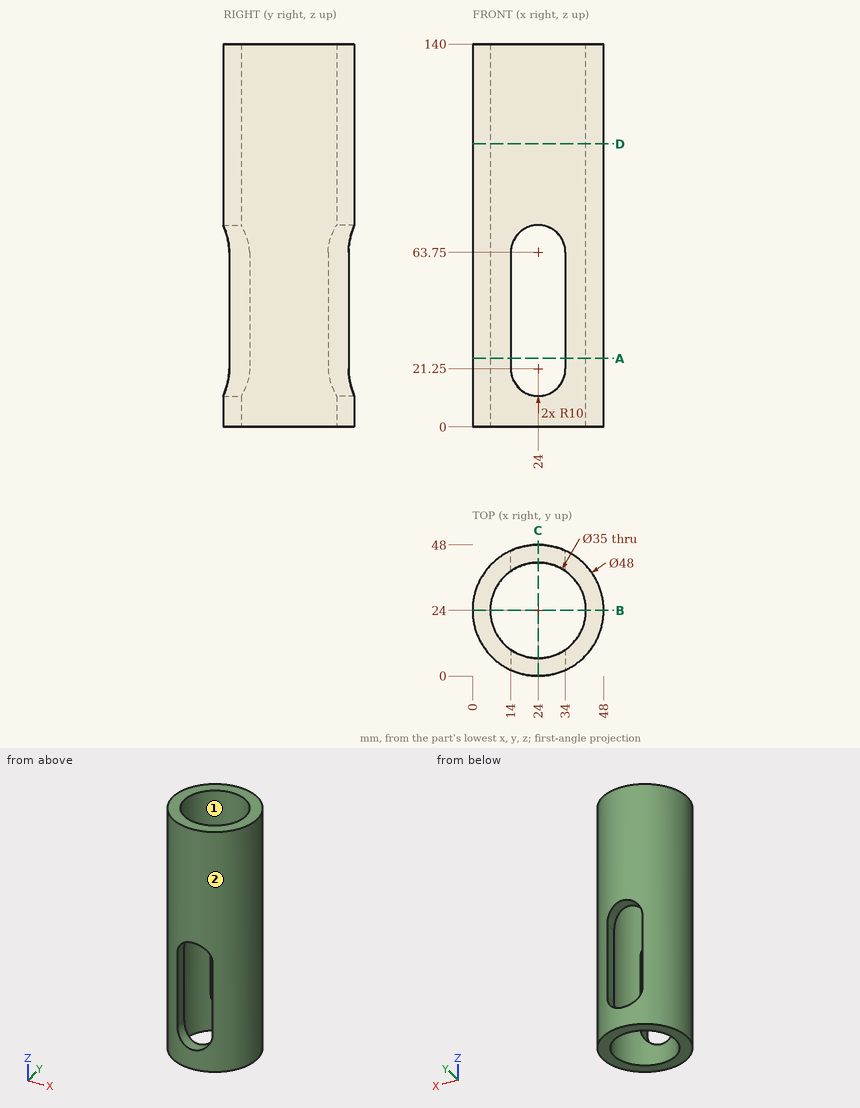
The figure shows three views and two pictorial views of one solid part (mm, origin at its lowest corner). Answer the questions. Coordinates: 2 decimals unless noted, no trailing zeros. Write each loop counter-clockwise with the first axis right and the second up, starting at its lowest first coordinate (ties: lowest second). Pieces come first, ordered by that corner, then holes.
1. The part is cut by section C-C, the plane x = 24. Write down the section's boundary in (y, z).
Results list:
outline: (0, 0) - (6.5, 0) - (6.5, 11.25) - (0, 11.25) - close; (0, 73.75) - (6.5, 73.75) - (6.5, 140) - (0, 140) - close; (41.5, 0) - (48, 0) - (48, 11.25) - (41.5, 11.25) - close; (41.5, 73.75) - (48, 73.75) - (48, 140) - (41.5, 140) - close
2. The part is cut by section B-B, the plane y = 24. Write down the section's boundary in (x, z).
Results list:
outline: (0, 0) - (6.5, 0) - (6.5, 140) - (0, 140) - close; (41.5, 0) - (48, 0) - (48, 140) - (41.5, 140) - close
3. Flat-ended cylindrical pins translate along their axes: pin 1 (2 mm diameter, centred on y = 5.5, z = 42, fed in from +X); pin 2 (4 mm diameter, centred on y = 40.5, z = 113, fed in from -X); pin 3 (1.5 mm diameter, centred on y = 33.5, z = 77, fed in from +X). Find the tip coordinate at first contact, or state that the pin passes through.
Results list:
pin 1: stops at x = 40.42
pin 2: stops at x = 4.88
pin 3: stops at x = 46.35
4. The part is cut by section D-D, the plane z = 103.5. Write down the section's boundary in (x, y).
Results list:
outline: circle Ø48 at (24, 24); hole circle Ø35 at (24, 24)
5. The part is cut by section A-A, the plane z = 25. Write down the section's boundary in (x, y).
Results list:
outline: (14, 2.18) - (14, 9.64) arc R17.5 cw to (14, 38.36) - (14, 45.82) arc R24 ccw to start; (34, 2.18) arc R24 ccw to (34, 45.82) - (34, 38.36) arc R17.5 cw to (34, 9.64) - close
6. For a pull along X with two mould halves and no side action, classify the marked faces 1 and 2 as +X half, -X half, draft (parallel to the pull), parting line (faces both ways), or undercut.
Results list:
face 1: undercut
face 2: parting line
7. Consider line 1 along Y through (x, z) = (24, 82); line 2 along X through (y, z) = (21, 131); line 3 along X through (y, z) = (28.5, 133). Determine where each line is inside the solid, lowest interval first.
Results list:
line 1: y = 0 to 6.5, 41.5 to 48
line 2: x = 0.19 to 6.76, 41.24 to 47.81
line 3: x = 0.43 to 7.09, 40.91 to 47.57
